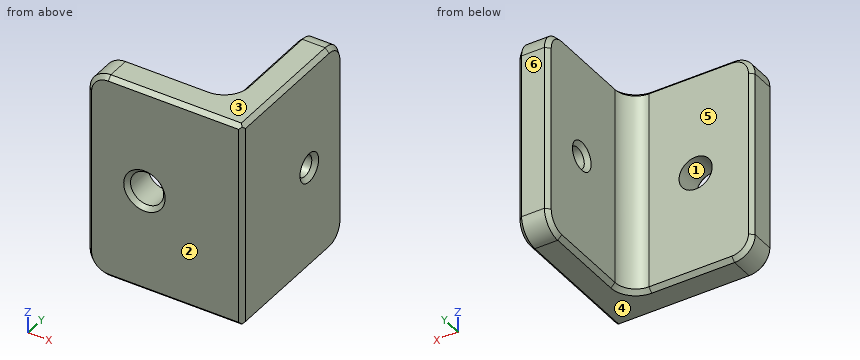
from build123d import *

# Parameters (mm, degrees)
SKETCH_1_W          = 15
SKETCH_1_H          = 20
EXTRUDE_1_DEPTH     = 3
SKETCH_2_R          = 1.6
CUT_EXTRUDE_1_DEPTH = 3
SKETCH_3_W          = 3
SKETCH_3_H          = 20
EXTRUDE_2_DEPTH     = 12
FILLET_1_R          = 2
SKETCH_4_R          = 1
CUT_EXTRUDE_2_DEPTH = 10
FILLET_2_R          = 2
CHAMFER_1_SIZE      = 0.4
CHAMFER_2_SIZE      = 0.4
CHAMFER_3_SIZE      = 0.4


with BuildPart() as part:
    # 草图1 → 凸台-拉伸1 (new body)
    with BuildSketch(Plane(origin=(0, 0, 0), x_dir=(1, 0, 0), z_dir=(0, 1, 0))):
        with Locations((7.5, 10)):
            Rectangle(SKETCH_1_W, SKETCH_1_H)
    extrude(amount=EXTRUDE_1_DEPTH)

    # 草图2 → 切除-拉伸1 (cut)
    with BuildSketch(Plane(origin=(0, 3, 0), x_dir=(1, 0, 0), z_dir=(0, 1, 0))):
        with Locations(Location((5.5, 10, 0), (0, 0, 270))):
            Circle(SKETCH_2_R)
    extrude(amount=-CUT_EXTRUDE_1_DEPTH, mode=Mode.SUBTRACT)

    # 草图3 → 凸台-拉伸2 (add)
    with BuildSketch(Plane(origin=(0, 3, 0), x_dir=(1, 0, 0), z_dir=(0, 1, 0))):
        with Locations((13.5, 10)):
            Rectangle(SKETCH_3_W, SKETCH_3_H)
    extrude(amount=EXTRUDE_2_DEPTH)

    # 圆角1
    fillet_1_edges = [part.edges().sort_by_distance(p)[0] for p in [
        (12, 3, -10),
    ]]
    fillet(fillet_1_edges, radius=FILLET_1_R)

    # 草图4 → 切除-拉伸2 (cut)
    with BuildSketch(Plane.ZY.offset(-12)):
        with Locations((-10, 10)):
            Circle(SKETCH_4_R)
    extrude(amount=-CUT_EXTRUDE_2_DEPTH, mode=Mode.SUBTRACT)

    # 圆角2
    fillet_2_edges = [part.edges().sort_by_distance(p)[0] for p in [
        (13.5, 15, -20),
        (13.5, 15, 0),
        (0, 1.5, -20),
        (0, 1.5, 0),
    ]]
    fillet(fillet_2_edges, radius=FILLET_2_R)

    # 倒角1
    chamfer_1_edges = [part.edges().sort_by_distance(p)[0] for p in [
        (5.5, 0, -11.6),
        (8.5, 0, -20),
        (8.5, 0, 0),
        (15, 0, -10),
        (0, 0, -10),
        (0.585786438, 0, -19.414213562),
        (0.585786438, 0, -0.585786438),
    ]]
    chamfer(chamfer_1_edges, length=CHAMFER_1_SIZE)

    # 倒角2
    chamfer_2_edges = [part.edges().sort_by_distance(p)[0] for p in [
        (15, 15, -10),
        (15, 6.7, -20),
        (15, 6.7, 0),
        (15, 14.414213562, -0.585786438),
        (15, 14.414213562, -19.414213562),
    ]]
    chamfer(chamfer_2_edges, length=CHAMFER_2_SIZE)

    # 倒角3
    chamfer_3_edges = [part.edges().sort_by_distance(p)[0] for p in [
        (6, 3, -20),
        (11.414213562, 3.585786438, 0),
        (11.414213562, 3.585786438, -20),
        (15, 10, -11),
        (12, 10, -11),
        (12, 15, -10),
        (12, 9, -20),
        (12, 9, 0),
        (12, 14.414213562, -0.585786438),
        (12, 14.414213562, -19.414213562),
        (6, 3, 0),
        (0, 3, -10),
        (0.585786438, 3, -19.414213562),
        (0.585786438, 3, -0.585786438),
    ]]
    chamfer(chamfer_3_edges, length=CHAMFER_3_SIZE)


solid = part.part
Read the model definition and answer for the solid it produces. Units are mm, in the model's axes. Face numbers are marked on the shaded views. A direction names the side the tool comes from. Round coordinates to 2 decimals unless told otherwise and drop trailing zeros. Order: outer loops, then holes, each group sorted by start corner. A loop starts at its lowest first (then second) coordinate and runs counter-clockwise, first axis right, second up.
1) The mould has two halves that part along Z. Classify the marked faces 1, 2, 3 and 4: released by +Z, released by -Z, zero draft, split by the parting line, or undercut.
2) Straight lines are drawn through the part: L1, parallel to X at y = 2.5, z = -10; L2, parallel to Y at x = 14.1, z = -10; L3, parallel to X at y = 8.5, z = -3.75. For each, find the intervals that lie inside material, in ascending order.
3) The part is cut by section B-B on y = 10. Write down the section's boundary in (x, z).
4) The part is cut by section C-C on x = 12.75. Write down the section's boundary in (y, z).
5) The part is cut by section D-D on y = 1.75. Write down the section's boundary in (x, z).
6) For the marked faces 5 and 6, determine the directions among +Z, -Z, +X, -X, +Y, -Y from which every point of the face is accessible in a straight line to the end or side of a thin tool.
7) Flat-ended cylindrical pins translate along their axes: pin 1 (1.2 mm diameter, centred on y = 10, z = -10, fed in from +X); pin 2 (1 mm diameter, centred on y = 7.5, z = -4.5, fed in from -X); pin 3 (6 mm diameter, centred on x = 11, y = 9.5, fed in from +Z); pin 4 (3 mm diameter, centred on x = 6.5, z = -14, fed in from +Y). Find the tip coordinate at first contact, or state that the pin passes through.
8) The part is cut by section A-A on z = -10. Write down the section's boundary in (x, y).
Resolved:
1. face 1: undercut
1. face 2: zero draft
1. face 3: released by +Z
1. face 4: released by -Z
2. L1: x = 0 to 3.9, 7.1 to 15
2. L2: y = 0 to 9, 11 to 15
2. L3: x = 12 to 15
3. outline: (12, -19.6) - (12.4, -20) - (14.6, -20) - (15, -19.6) - (15, -11.4) - (14.6, -11) - (12.4, -11) - (12, -11.4) - close; (12, -8.6) - (12.4, -9) - (14.6, -9) - (15, -8.6) - (15, -0.4) - (14.6, 0) - (12.4, 0) - (12, -0.4) - close
4. outline: (0, -19.6) - (0.4, -20) - (13, -20) arc R2 ccw to (15, -18) - (15, -2) arc R2 ccw to (13, 0) - (0.4, 0) - (0, -0.4) - close; hole circle Ø2 at (10, -10)
5. outline: (0, -18) arc R2 ccw to (2, -20) - (14.6, -20) - (15, -19.6) - (15, -0.4) - (14.6, 0) - (2, 0) arc R2 ccw to (0, -2) - close; hole circle Ø3.2 at (5.5, -10)
6. face 5: +Z, -Z, -X, +Y
6. face 6: +Z, -Z, +X, -X, +Y
7. pin 1: passes through
7. pin 2: stops at x = 12
7. pin 3: stops at z = 0
7. pin 4: stops at y = 3
8. outline: (0, 0.4) - (0.4, 0) - (3.5, 0) - (3.9, 0.4) - (3.9, 3) - (0.4, 3) - (0, 2.6) - close; (7.1, 0.4) - (7.5, 0) - (14.6, 0) - (15, 0.4) - (15, 8.6) - (14.6, 9) - (12.4, 9) - (12, 8.6) - (12, 5) arc R2 cw to (10, 3) - (7.1, 3) - close; (12, 11.4) - (12.4, 11) - (14.6, 11) - (15, 11.4) - (15, 14.6) - (14.6, 15) - (12.4, 15) - (12, 14.6) - close
